For this review, take the finished solid that the model builds, in its own axes (mm). A direction names the side the tool comes from. Coordinates: 2 decimals unless noted, no trailing zeros. Write each loop counter-clockwise with the first axis right and the second up, starting at its lowest first coordinate (ties: lowest second). Pieces come first, ordered by that corner, then holes. Notation, with made-up numbers: (40.5, 45) -> (49.5, 45) arc R10 ccw to (49.5, 59) -> close; hole circle Ø9 at (-33, -39.75). An arc over 180 degrees is marked (long way). Put each result on its own line as item: value. Start each with the question number.
Item 1: Consider section B-B on y = -2.5. Give the boundary of the cut face in (x, z), and give its area (3 significant figures).
Item 2: Insertion check: P1, Ø6.5, axis at x = 51, z = 34, coming from the -Y side; P2, Ø12, axis at x = 61.91, z = 61.91, coming from the +Y side; P3, Ø12, axis at x = -61.91, z = -61.91, coming from the -Y side. Each pin has a flat end and moves straight along its axis. Give the tip position at first contact, or say it passes through.
Item 3: To check wall thickness, follow L1, parallel to Z at x = 1, y = 3.75; L2, parallel to Z at x = 28, y = 2.75; L3, parallel to Z at x = 8, y = 0.25. State the ranges of each line that lie inside material, in increasing order.
Item 4: Consider section C-C on x = 19. Give the boundary of the cut face in (y, z) (1 decimal).
Item 5: Consider section A-A on x = 50.8. Give the boundary of the cut face in (y, z) (1 decimal).
Item 6: For faces 1 (the cylindrical face through (0.28, -2.42, -15.88)), 2 (the cylindrical face through (-0.867, 1.366, 67.891)), 3 (the flat face through (-74.612, 0, 1)), list the 3-axis set-ups (+Z, -Z, +X, -X, +Y, -Y) from which the entire face can be reached by the end or side of a thin tool; tool diameter is ignored.
Item 7: The part is to be moulded in two halves that separate along Z. For faces 4 (the conical face through (69.876, -5.677, -70.053)), 5 (the cylindrical face through (56.15, -2.42, 29.89)), 6 (the conical face through (69.9, 5.7, 70)), say which applies: +Z half, -Z half, draft (parallel to the pull), parting line (faces both ways), or undercut.
```python
from build123d import *

# Parameters (mm, degrees)
BOSS_EXTRUDE1_DEPTH      = 76.2
BOSS_EXTRUDE1_DEPTH_BACK = 76.2
SKETCH3_W                = 152.4
SKETCH3_H                = 11.90625
SKETCH8_OUTSIDE_W        = 197.57
SKETCH8_OUTSIDE_H        = 197.57
CUT_EXTRUDE2_DEPTH       = 109.41881197
CHAMFER1_SIZE            = 1.5875
PEN_SLOT_CUT_DEPTH       = 6.35
PEN_SLOT_FILLET_R        = 6.35
HOLE1_D                  = 4.7625
HOLE1_CBORE_D            = 12.7
HOLE1_CBORE_DEPTH        = 6.35
SKETCH6_R                = 6.746875
CUT_EXTRUDE1_DEPTH       = 1.524
BASE_CHAMFERS_SIZE       = 0.79375


# Some blends are built 0.0001 mm under size
with BuildPart() as part:
    # Sketch3 → Boss-Extrude1 (new, two sides: drawn at the far end of the back side and taken through both)
    with BuildSketch(Plane(origin=(0, 0, 0), x_dir=(0, 0, -1), z_dir=(1, 0, 0)).offset(-BOSS_EXTRUDE1_DEPTH_BACK)):
        Rectangle(SKETCH3_W, SKETCH3_H)
    extrude(amount=BOSS_EXTRUDE1_DEPTH + BOSS_EXTRUDE1_DEPTH_BACK)

    # Sketch8 outside → Cut-Extrude2 (cut, through all)
    with BuildSketch(Plane.XZ.offset(5.953125)):
        Rectangle(SKETCH8_OUTSIDE_W, SKETCH8_OUTSIDE_H)
        with BuildLine():
            Line((-61.9125, -74.6125), (61.9125, -74.6125))
            ThreePointArc((61.9125, -74.6125), (70.892756121, -70.892756121), (74.6125, -61.9125))
            Line((74.6125, -61.9125), (74.6125, 61.9125))
            ThreePointArc((74.6125, 61.9125), (70.892756121, 70.892756121), (61.9125, 74.6125))
            Line((61.9125, 74.6125), (-61.9125, 74.6125))
            ThreePointArc((-61.9125, 74.6125), (-70.892756121, 70.892756121), (-74.6125, 61.9125))
            Line((-74.6125, 61.9125), (-74.6125, -61.9125))
            ThreePointArc((-74.6125, -61.9125), (-70.892756121, -70.892756121), (-61.9125, -74.6125))
        make_face(mode=Mode.SUBTRACT)
    extrude(amount=-CUT_EXTRUDE2_DEPTH, mode=Mode.SUBTRACT)

    # Chamfer1
    chamfer1_edges = [part.edges().sort_by_distance(p)[0] for p in [
        (-74.6125, 5.953125, 0),
        (-70.892756121, 5.953125, -70.892756121),
        (0, 5.953125, -74.6125),
        (70.892756121, 5.953125, -70.892756121),
        (74.6125, 5.953125, 0),
        (70.892756121, 5.953125, 70.892756121),
        (0, 5.953125, 74.6125),
        (-70.892756121, 5.953125, 70.892756121),
        (-70.892756121, -5.953125, -70.892756121),
        (-74.6125, -5.953125, 0),
        (-70.892756121, -5.953125, 70.892756121),
        (0, -5.953125, 74.6125),
        (70.892756121, -5.953125, 70.892756121),
        (74.6125, -5.953125, 0),
        (70.892756121, -5.953125, -70.892756121),
        (0, -5.953125, -74.6125),
    ]]
    chamfer(chamfer1_edges, length=CHAMFER1_SIZE)

    # Pen Slot Sketch → Pen Slot Cut (cut)
    with BuildSketch(Plane(origin=(0, 5.953125, 0), x_dir=(1, 0, 0), z_dir=(0, 1, 0))):
        with BuildLine():
            Line((-61.9125, -53.975), (61.9125, -53.975))
            ThreePointArc((61.9125, -53.975), (69.85, -61.9125), (61.9125, -69.85))
            Line((61.9125, -69.85), (-61.9125, -69.85))
            ThreePointArc((-61.9125, -69.85), (-69.85, -61.9125), (-61.9125, -53.975))
        make_face()
    extrude(amount=-PEN_SLOT_CUT_DEPTH, mode=Mode.SUBTRACT)

    # Pen Slot Fillet
    pen_slot_fillet_edges = [part.edges().sort_by_distance(p)[0] for p in [
        (0, -0.396875, 53.975),
        (69.85, -0.396875, 61.9125),
        (0, -0.396875, 69.85),
        (-69.85, -0.396875, 61.9125),
    ]]
    fillet(pen_slot_fillet_edges, radius=PEN_SLOT_FILLET_R - 0.0001)  # a hair under: the kernel refuses the full size

    # Hole1 (through all)
    with Locations(Plane(origin=(-50.8, -5.953125, 33.30776944), x_dir=(0, 0, -1), z_dir=(0, -1, 0))):
        with Locations((0, 0), (0, 101.6), (55.531312028, 50.8)):
            CounterBoreHole(HOLE1_D / 2, HOLE1_CBORE_D / 2, HOLE1_CBORE_DEPTH)

    # Sketch6 → Cut-Extrude1 (cut)
    with BuildSketch(Plane(origin=(0, -5.953125, 0), x_dir=(-1, 0, 0), z_dir=(0, -1, 0))):
        with Locations(Location((-61.9125, 61.9125, 0), (0, 0, 90))):
            Circle(SKETCH6_R)
        with Locations(Location((61.9125, 61.9125, 0), (0, 0, 90))):
            Circle(SKETCH6_R)
        with Locations(Location((61.9125, -61.9125, 0), (0, 0, 90))):
            Circle(SKETCH6_R)
        with Locations(Location((-61.9125, -61.9125, 0), (0, 0, 90))):
            Circle(SKETCH6_R)
    extrude(amount=-CUT_EXTRUDE1_DEPTH, mode=Mode.SUBTRACT)

    # Chamfer2
    # the kernel refuses this chamfer: 0.396875 mm, written as the material it takes off along each edge
    with BuildSketch(Plane(origin=(-61.9125, 5.953125, 61.9125), x_dir=(0, 0, 1), z_dir=(1, 0, 0))) as chamfer2_piece_1:
        with BuildLine():
            Line((7.853310099, 0.481064901), (8.418564901, -0.084189901))
            Line((8.418564901, -0.084189901), (8.418564901, -0.143721151))
            ThreePointArc((8.418564901, -0.143721151), (8.178032451, -0.05953125), (7.9375, -0.05953125))
            Line((7.9375, -0.05953125), (7.87796875, 0))
            ThreePointArc((7.87796875, 0), (7.87796875, 0.240532451), (7.793778849, 0.481064901))
            Line((7.793778849, 0.481064901), (7.853310099, 0.481064901))
        make_face()
    revolve(axis=Axis((-61.9125, 5.953125, 61.9125), (0, -1, 0)), revolution_arc=180, mode=Mode.SUBTRACT)
    with BuildSketch(Plane(origin=(61.9125, 5.953125, 69.85), x_dir=(0, 0.17238737169530088, 0.9850292351397425), z_dir=(-1, 0, 0))) as chamfer2_piece_2:
        with BuildLine():
            Line((0.488376267, 0), (-0.165859028, -0.459349716))
            Line((-0.165859028, -0.459349716), (-0.224499049, -0.44908728))
            ThreePointArc((-0.224499049, -0.44908728), (-0.100104779, -0.22666906), (-0.058640022, 0.010262436))
            Line((-0.058640022, 0.010262436), (0.010262436, 0.058640022))
            ThreePointArc((0.010262436, 0.058640022), (0.247193932, 0.017175265), (0.498638703, 0.058640022))
            Line((0.498638703, 0.058640022), (0.488376267, 0))
        make_face()
    extrude(amount=123.825, mode=Mode.SUBTRACT)
    with BuildSketch(Plane(origin=(61.9125, 5.953125, 61.9125), x_dir=(0, 0, -1), z_dir=(-1, 0, 0))) as chamfer2_piece_3:
        with BuildLine():
            Line((8.418564901, -0.084189901), (7.853310099, 0.481064901))
            Line((7.853310099, 0.481064901), (7.793778849, 0.481064901))
            ThreePointArc((7.793778849, 0.481064901), (7.87796875, 0.240532451), (7.87796875, 0))
            Line((7.87796875, 0), (7.9375, -0.05953125))
            ThreePointArc((7.9375, -0.05953125), (8.178032451, -0.05953125), (8.418564901, -0.143721151))
            Line((8.418564901, -0.143721151), (8.418564901, -0.084189901))
        make_face()
    revolve(axis=Axis((61.9125, 5.953125, 61.9125), (0, -1, 0)), revolution_arc=180, mode=Mode.SUBTRACT)
    with BuildSketch(Plane(origin=(-61.9125, 5.953125, 53.975), x_dir=(0, -0.9850292351397427, 0.17238737169529986), z_dir=(1, 0, 0))) as chamfer2_piece_4:
        with BuildLine():
            Line((0.488376267, 0), (-0.165859028, 0.459349716))
            Line((-0.165859028, 0.459349716), (-0.224499049, 0.44908728))
            ThreePointArc((-0.224499049, 0.44908728), (-0.100104779, 0.22666906), (-0.058640022, -0.010262436))
            Line((-0.058640022, -0.010262436), (0.010262436, -0.058640022))
            ThreePointArc((0.010262436, -0.058640022), (0.247193932, -0.017175265), (0.498638703, -0.058640022))
            Line((0.498638703, -0.058640022), (0.488376267, 0))
        make_face()
    extrude(amount=123.825, mode=Mode.SUBTRACT)
    with BuildSketch(Plane(origin=(61.9125, -5.953125, 61.9125), x_dir=(0, 0, -1), z_dir=(-1, 0, 0))) as chamfer2_piece_5:
        with BuildLine():
            Line((7.227939901, 0.084189901), (6.662685099, -0.481064901))
            Line((6.662685099, -0.481064901), (6.603153849, -0.481064901))
            ThreePointArc((6.603153849, -0.481064901), (6.68734375, -0.240532451), (6.68734375, 0))
            Line((6.68734375, 0), (6.746875, 0.05953125))
            ThreePointArc((6.746875, 0.05953125), (6.987407451, 0.05953125), (7.227939901, 0.143721151))
            Line((7.227939901, 0.143721151), (7.227939901, 0.084189901))
        make_face()
    revolve(axis=Axis((61.9125, -5.953125, 61.9125), (0, -1, 0)), mode=Mode.SUBTRACT)
    with BuildSketch(Plane(origin=(-61.9125, -5.953125, 61.9125), x_dir=(0, 0, -1), z_dir=(-1, 0, 0))) as chamfer2_piece_6:
        with BuildLine():
            Line((7.227939901, 0.084189901), (6.662685099, -0.481064901))
            Line((6.662685099, -0.481064901), (6.603153849, -0.481064901))
            ThreePointArc((6.603153849, -0.481064901), (6.68734375, -0.240532451), (6.68734375, 0))
            Line((6.68734375, 0), (6.746875, 0.05953125))
            ThreePointArc((6.746875, 0.05953125), (6.987407451, 0.05953125), (7.227939901, 0.143721151))
            Line((7.227939901, 0.143721151), (7.227939901, 0.084189901))
        make_face()
    revolve(axis=Axis((-61.9125, -5.953125, 61.9125), (0, -1, 0)), mode=Mode.SUBTRACT)
    with BuildSketch(Plane(origin=(-61.9125, -5.953125, -61.9125), x_dir=(0, 0, -1), z_dir=(-1, 0, 0))) as chamfer2_piece_7:
        with BuildLine():
            Line((7.227939901, 0.084189901), (6.662685099, -0.481064901))
            Line((6.662685099, -0.481064901), (6.603153849, -0.481064901))
            ThreePointArc((6.603153849, -0.481064901), (6.68734375, -0.240532451), (6.68734375, 0))
            Line((6.68734375, 0), (6.746875, 0.05953125))
            ThreePointArc((6.746875, 0.05953125), (6.987407451, 0.05953125), (7.227939901, 0.143721151))
            Line((7.227939901, 0.143721151), (7.227939901, 0.084189901))
        make_face()
    revolve(axis=Axis((-61.9125, -5.953125, -61.9125), (0, -1, 0)), mode=Mode.SUBTRACT)
    with BuildSketch(Plane(origin=(61.9125, -5.953125, -61.9125), x_dir=(0, 0, -1), z_dir=(-1, 0, 0))) as chamfer2_piece_8:
        with BuildLine():
            Line((7.227939901, 0.084189901), (6.662685099, -0.481064901))
            Line((6.662685099, -0.481064901), (6.603153849, -0.481064901))
            ThreePointArc((6.603153849, -0.481064901), (6.68734375, -0.240532451), (6.68734375, 0))
            Line((6.68734375, 0), (6.746875, 0.05953125))
            ThreePointArc((6.746875, 0.05953125), (6.987407451, 0.05953125), (7.227939901, 0.143721151))
            Line((7.227939901, 0.143721151), (7.227939901, 0.084189901))
        make_face()
    revolve(axis=Axis((61.9125, -5.953125, -61.9125), (0, -1, 0)), mode=Mode.SUBTRACT)

    # Base Chamfers
    base_chamfers_edges = [part.edges().sort_by_distance(p)[0] for p in [
        (0, -5.953125, -15.873542588),
        (50.8, -5.953125, 39.65776944),
        (-50.8, -5.953125, 39.65776944),
    ]]
    chamfer(base_chamfers_edges, length=BASE_CHAMFERS_SIZE)


solid = part.part
```
Return value:
1. outline: (-74.61, -61.91) arc R12.7 ccw to (-61.91, -74.61) -> (61.91, -74.61) arc R12.7 ccw to (74.61, -61.91) -> (74.61, 61.91) arc R12.7 ccw to (61.91, 74.61) -> (-61.91, 74.61) arc R12.7 ccw to (-74.61, 61.91) -> close; hole circle Ø12.7 at (-50.8, 33.31); hole circle Ø12.7 at (0, -22.22); hole circle Ø12.7 at (50.8, 33.31)
1. area: 21,700 mm^2
2. P1: y = 0.4
2. P2: y = 1.39
2. P3: y = -4.43
3. L1: -74.61 to -24.38, -20.06 to 54.37, 69.46 to 74.61
3. L2: -74.61 to 54.84, 68.98 to 74.61
3. L3: -74.61 to 57.53, 66.29 to 74.61
4. outline: (-6, -73) -> (-4.4, -74.6) -> (4.4, -74.6) -> (6, -73) -> (6, 53.6) -> (5.5, 54) arc R6.3 cw to (-0.4, 60.3) -> (-0.4, 63.5) arc R6.3 cw to (5.5, 69.8) -> (6, 70.2) -> (6, 73) -> (4.4, 74.6) -> (-4.4, 74.6) -> (-6, 73) -> close
5. outline: (-6, -73) -> (-4.4, -74.6) -> (4.4, -74.6) -> (6, -73) -> (6, 30.9) -> (0.4, 30.9) -> (0.4, 27) -> (-5.2, 27) -> (-6, 26.2) -> close; (-6, 40.5) -> (-5.2, 39.7) -> (0.4, 39.7) -> (0.4, 35.7) -> (6, 35.7) -> (6, 53.6) -> (5.5, 54) arc R6.3 cw to (-0.4, 60.3) -> (-0.4, 63.5) arc R6.3 cw to (5.5, 69.8) -> (6, 70.2) -> (6, 73) -> (4.4, 74.6) -> (-4.4, 74.6) -> (-6, 73) -> close
6. face 1: -Y
6. face 2: +Y
6. face 3: +Z, -Z, -X, +Y, -Y
7. face 4: -Z half
7. face 5: undercut
7. face 6: +Z half
